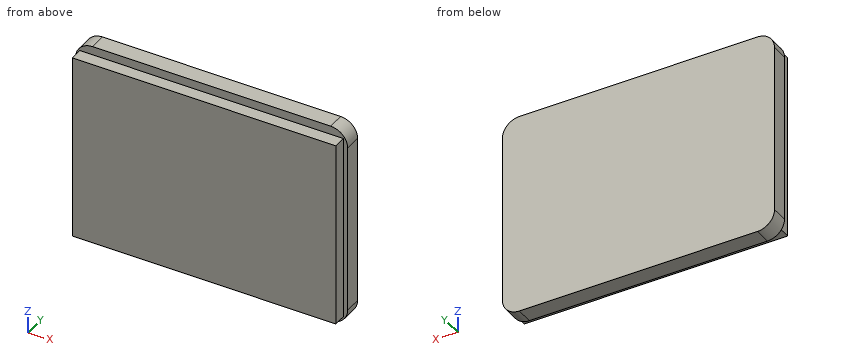
from build123d import *

# Parameters (mm, degrees)
F0_W     = 160
F0_H     = 120
F1_DEPTH = 10
F2_R     = 10
F3_W     = 154.9
F3_H     = 109.9
F4_DEPTH = 7.5


with BuildPart() as f1:
    # F0 (on Front) → F1 (new body)
    with BuildSketch(Plane.XZ):
        with Locations((5.032664, 11.062619)):
            Rectangle(F0_W, F0_H)
    extrude(amount=F1_DEPTH)

    # F2
    f2_edges = [f1.edges().sort_by_distance(p)[0] for p in [
        (-74.967336, -5, 71.062619),
        (-74.967336, -5, -48.937381),
        (85.032664, -5, 71.062619),
        (85.032664, -5, -48.937381),
    ]]
    fillet(f2_edges, radius=F2_R)

    # F3 (on face) → F4 (join)
    with BuildSketch(Plane.XZ.offset(10)):
        with Locations((5.032664, 11.062619)):
            Rectangle(F3_W, F3_H)
    extrude(amount=F4_DEPTH)


solid = f1.part
Design review of the part built by this model. Coordinates are the model's own, in mm. Round coordinates to 2 decimals unless told otherwise and drop trailing zeros. Write each loop counter-clockwise with the first axis right and the second up, starting at its lowest first coordinate (ties: lowest second). Pieces come first, ordered by that corner, then holes.
Item 1: Consider section B-B on y = -13.5. Give the boundary of the cut face in (x, z).
Item 2: Consider section A-A on x = 61. Give the boundary of the cut face in (y, z).
Item 3: Wall thickness on L1, parallel to X at y = -11.5, z = -10.5; L2, parallel to Z at x = -64, y = -14: over which ranges is each line inside the solid? List them lowest first.
Item 4: For pin 1 Ø8 at (y, z) = (-12, 27) entering from -X; pin 2 Ø2 at (y, z) = (-15, -3) entering from +X; pin 3 Ø8 at (x, y) = (-12.5, -15.5) entering from -Z; pin 4 Ø4 at (x, y) = (17, -13.5) entering from +Z, all flat-tipped, find the tip position at first contact; note any pin that passes through.
Check values:
1. outline: (-72.42, -43.89) - (82.48, -43.89) - (82.48, 66.01) - (-72.42, 66.01) - close
2. outline: (-17.5, -43.89) - (-10, -43.89) - (-10, -48.94) - (0, -48.94) - (0, 71.06) - (-10, 71.06) - (-10, 66.01) - (-17.5, 66.01) - close
3. L1: x = -72.42 to 82.48
3. L2: z = -43.89 to 66.01
4. pin 1: stops at x = -74.97
4. pin 2: stops at x = 82.48
4. pin 3: stops at z = -43.89
4. pin 4: stops at z = 66.01
